from build123d import *


with BuildPart() as part:
    # Sketch1 → Revolve1 (revolve)
    with BuildSketch(Plane.XY):
        with BuildLine():
            Line((4.07, 9.6), (2, 9.6))
            Line((2, 9.6), (2, -0.75))
            Line((2, -0.75), (4.445, -0.75))
            Line((4.445, -0.75), (4.445, -0.125))
            ThreePointArc((4.445, -0.125), (4.481611652, -0.036611652), (4.57, 0))
            Line((4.57, 0), (7.1, 0))
            Line((7.1, 0), (7.1, 0.75))
            Line((7.1, 0.75), (6.464541397, 0.75))
            ThreePointArc((6.464541397, 0.75), (6.380092621, 0.782840333), (6.340017059, 0.864105532))
            Line((6.340017059, 0.864105532), (5.671290647, 8.507683404))
            ThreePointArc((5.671290647, 8.507683404), (5.551063963, 8.751479001), (5.297717635, 8.85))
            Line((5.297717635, 8.85), (5.043170913, 8.85))
            Line((5.043170913, 8.85), (5.043170913, 8.6))
            Line((5.043170913, 8.6), (4.445, 8.6))
            Line((4.445, 8.6), (4.445, 9.225))
            ThreePointArc((4.445, 9.225), (4.335165043, 9.490165043), (4.07, 9.6))
        make_face()
    revolve(axis=Axis((0, 9.60267581, 0), (0, -1, 0)))


solid = part.part
Geometry check sheet. Reference: the model listing, model coordinates, mm. A direction names the side the tool comes from. Round coordinates to 2 decimals unless told otherwise and drop trailing zeros. Loops run counter-clockwise (first coordinate to the right, second up) from the corner with the lowest first, then second, coordinate; pieces in that order, holes last.
Item 1: Thickness scan on line 1 (Z direction, x = 0, y = 8.8) (3 decimals); line 2 (Y direction, x = -2.75, z = -4); line 3 (Y direction, x = 5.5, z = -4.25). Record the ranges inside material, lowest first.
Item 2: Mould release check, pull along Z, two halves, no side actions. Record for faces 4 (the cylindrical face through (0, 4, -2)), 5 (the conical face through (5.653, 5.589, 1.78)), 6 (the flat face through (1, 9.6, 2)): pulls with the +Z half, pulls with the -Z half, needs draft (parallel to the pull), parting line crosses it, or undercut.
Item 3: Cross-section at C-C on y = 4.5. Record the boundary of the cut face in (x, z), then the cut area to 3 significant figures.
Item 4: Gauge pin test, flat ends, axial feed: pin 1 (2 mm diameter, centred on x = 4.5, y = 5.5, fed in from -Z); pin 2 (6 mm diameter, centred on x = 0, z = 0, fed in from +Y); pin 3 (1 mm diameter, centred on x = 3.5, y = 3.5, fed in from -Z); pin 4 (1 mm diameter, centred on x = 1.5, y = 0.5, fed in from +Z). Record the tip position at first contact, or that the pin passes through.
Item 5: Access from +Z, -Z, +X, -X, +Y, -Y to the whole of each face (thin tool, end or side, straight path). Record for faces 1 (the cylindrical face through (-0.92, 0.38, 7.04)), 2 (the flat face through (3, 0.75, -6)), 3 (the flat face through (0, 0, -5)).
Answer sheet:
1. line 1: z = -5.485 to -5.043, -4.445 to -2, 2 to 4.445, 5.043 to 5.485
1. line 2: y = 0 to 8.6
1. line 3: y = 0 to 0.75
2. face 4: undercut
2. face 5: parting line crosses it
2. face 6: needs draft
3. outline: circle Ø12.04 at (0, 0); hole circle Ø4 at (0, 0)
3. area: 101 mm2
4. pin 1: stops at z = -4.8
4. pin 2: stops at y = 9.6
4. pin 3: stops at z = -5.33
4. pin 4: stops at z = 7.03
5. face 1: +Y, -Y
5. face 2: +Y
5. face 3: -Y
